```python
from build123d import *

# Parameters (mm, degrees)
EXTRUDE_1_DEPTH     = 1
SKETCH_2_R          = 1.15
CUT_EXTRUDE_1_DEPTH = 54.115440316
SKETCH_3_R          = 1.15
CUT_EXTRUDE_2_DEPTH = 54.115440316
SKETCH_4_W          = 5.2
SKETCH_4_H          = 5.2
EXTRUDE_2_DEPTH     = 1.7


with BuildPart() as part:
    # Эскиз1 → Бобышка-Вытянуть1 (new body)
    with BuildSketch(Plane(origin=(0, 0, 0), x_dir=(1, 0, 0), z_dir=(0, 1, 0))):
        Polygon((0, 0), (0, 18), (18, 18), (31.75, 27), (31.75, 32.5), (39.25, 32.5), (39.25, 17.8), (42, 17.8), (42, -5.2), (20, -5.2), (20, 0), align=None)
    extrude(amount=EXTRUDE_1_DEPTH)

    # Эскиз2 → Вырез-Вытянуть1 (cut, through all)
    with BuildSketch(Plane(origin=(0, 1, 0), x_dir=(1, 0, 0), z_dir=(0, 1, 0))):
        with Locations(Location((35.7, 29.15, 0), (0, 0, 270))):
            Circle(SKETCH_2_R)
    extrude(amount=-CUT_EXTRUDE_1_DEPTH, mode=Mode.SUBTRACT)

    # Эскиз3 → Вырез-Вытянуть2 (cut, through all)
    with BuildSketch(Plane(origin=(0, 1, 0), x_dir=(1, 0, 0), z_dir=(0, 1, 0))):
        with Locations(Location((25.55, -2.55, 0), (0, 0, 270))):
            Circle(SKETCH_3_R)
    extrude(amount=-CUT_EXTRUDE_2_DEPTH, mode=Mode.SUBTRACT)

    # Эскиз4 → Бобышка-Вытянуть2 (add)
    with BuildSketch(Plane.XZ):
        with Locations((38.4, -9)):
            Rectangle(SKETCH_4_W, SKETCH_4_H)
    extrude(amount=EXTRUDE_2_DEPTH)


solid = part.part
```
Input: part model. Units: mm. Frame: model coordinates. A direction names the side the tool comes from. Give positions to 0.01 mm unless a question says otherwise; leave off trailing zeros. Order: outer loops, then holes, each group sorted by start corner. A loop starts at its lowest first (then second) coordinate and runs counter-clockwise, first axis right, second up. Notation, with made-up numbers: (14.5, 84.25) - (31.5, 84.25) arc R10 cw to (31.5, 100.25) - close; hole circle Ø4 at (-17, 37.25). An arc over 180 degrees is marked (long way). Use a Markdown table: item, result.
(1) Access query for faces 1 (the flat face through (38, -1, -11.6)), 2 (the flat face through (38, -1, -6.4)), 3 (the flat face through (40.6, 0.5, -17.8)), 4 (the flat face through (20, 0.5, 2.6)), 5 (the flat face through (8.9, 0.5, -18)). Directions: +Z, -Z, +X, -X, +Y, -Y. A direction counts if a zero-diameter tool reaches every point of the face in a straight line with its end or side. Return the directions, or none.
Computed values:
| item | result |
|---|---|
| face 1 | -Z, +X, -X, -Y |
| face 2 | +Z, +X, -X, -Y |
| face 3 | -Z, +X, +Y, -Y |
| face 4 | +Z, -X, +Y, -Y |
| face 5 | -Z, -X, +Y, -Y |
(2) Section query B-B (z = 2.55). Output: boundary loops of the cut face in (x, y).
Computed values:
| item | result |
|---|---|
| outline | (20, 0) - (24.4, 0) - (24.4, 1) - (20, 1) - close; (26.7, 0) - (42, 0) - (42, 1) - (26.7, 1) - close |
(3) Draft query along X for faces 6 (the flat face through (26, 1, -10)), 7 (the flat face through (35.8, -1, -9)), 8 (the cylindrical face through (24.53, 0.51, 3.08)). Return one class per face: released by +X, released by -X, zero draft, split by the parting line, or undercut.
Computed values:
| item | result |
|---|---|
| face 6 | zero draft |
| face 7 | released by -X |
| face 8 | undercut |
(4) Line query: line 1 (X direction, y = 0.25, z = -29.15); line 2 (Y direction, x = 26, z = -18); line 3 (X direction, y = 0.2, z = 2.55). Output: solid intervals per line, ascending. Write a range as from..to.
Computed values:
| item | result |
|---|---|
| line 1 | x = 31.75..34.55, 36.85..39.25 |
| line 2 | y = 0..1 |
| line 3 | x = 20..24.4, 26.7..42 |
(5) Section query A-A (z = -29.15). Output: boundary loops of the cut face in (x, y), then the cut area to 3 significant figures.
Computed values:
| item | result |
|---|---|
| outline | (31.75, 0) - (34.55, 0) - (34.55, 1) - (31.75, 1) - close; (36.85, 0) - (39.25, 0) - (39.25, 1) - (36.85, 1) - close |
| area | 5.20 mm2 |
(6) Pin query (flat end, axial travel): pin 1 (0.8 mm diameter, centred on y = 0.5, z = 1.5, fed in from -X); pin 2 (0.8 mm diameter, centred on y = 0.5, z = -28.5, fed in from -X); pin 3 (1.5 mm diameter, centred on x = 11.5, y = 0, fed in from -Z); pin 4 (1.8 mm diameter, centred on x = 35.7, z = -29.15, fed in from -Y). Return the tip coordinate at first contact, or that it passes through.
Computed values:
| item | result |
|---|---|
| pin 1 | stops at x = 20 |
| pin 2 | stops at x = 31.75 |
| pin 3 | stops at z = -18 |
| pin 4 | passes through |
(7) Section query D-D (x = 30.5). Output: boundary loops of the cut face in (y, z).
Computed values:
| item | result |
|---|---|
| outline | (0, -26.18) - (1, -26.18) - (1, 5.2) - (0, 5.2) - close |
(8) Section query C-C (y = -0.85). Output: boundary loops of the cut face in (x, z).
Computed values:
| item | result |
|---|---|
| outline | (35.8, -11.6) - (41, -11.6) - (41, -6.4) - (35.8, -6.4) - close |
